Source: three-view drawing plus pictorial views. Frame: mm from the lowest corner of the part. Give positions to 0.01 mm unless a question says otherwise; leave off trailing zeros. Write each loop counter-clockwise with the first axis right and the second up, starting at its lowest first coordinate (ties: lowest second). Pieces come first, ordered by that corner, then holes.
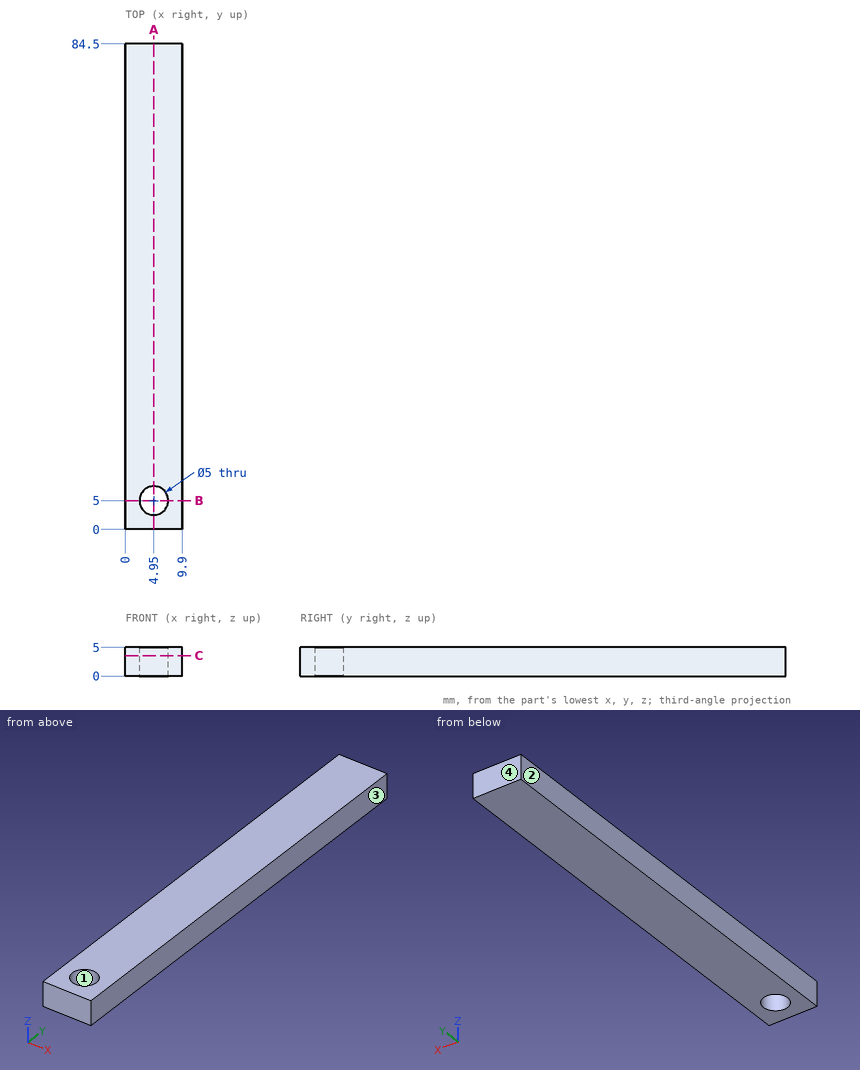
Q1. Ray query, line 1 along Y through (x, z) = (4.95, 1.1); line 2 along Y through (x, z) = (6.75, 3.9); line 3 along X through (y, z) = (6.5, 3.55). Return the intervals inside material, ascending.
Filled sheet:
line 1: y = 0 to 2.5, 7.5 to 84.5
line 2: y = 0 to 3.27, 6.73 to 84.5
line 3: x = 0 to 2.95, 6.95 to 9.9
Q2. Pin query (flat end, axial travel): P1, Ø1.5, axis at x = 7, y = 43.5, coming from the -Z side; P2, Ø4, axis at x = 4.95, y = 5, coming from the -Z side. Return the tip coordinate at first contact, or that it passes through.
Filled sheet:
P1: stops at z = 0
P2: passes through
Q3. Section B-B on y = 5. Output: boundary loops of the cut face in (x, z), plus the area to 3 significant figures.
Filled sheet:
outline: (0, 0) - (2.45, 0) - (2.45, 5) - (0, 5) - close; (7.45, 0) - (9.9, 0) - (9.9, 5) - (7.45, 5) - close
area: 24.5 mm2
Q4. Pull-direction query (X, two-part tool) for the marked faces 1, 2, 3 and 4; classes: released by +X, released by -X, zero draft, split by the parting line, or undercut.
Filled sheet:
face 1: undercut
face 2: released by -X
face 3: released by +X
face 4: zero draft
Q5. Section C-C on z = 3.55. Output: boundary loops of the cut face in (x, y), plus the area to 3 significant figures.
Filled sheet:
outline: (0, 0) - (9.9, 0) - (9.9, 84.5) - (0, 84.5) - close; hole circle Ø5 at (4.95, 5)
area: 817 mm2
Q6. Section A-A on x = 4.95. Output: boundary loops of the cut face in (y, z), plus the area to 4 significant figures.
Filled sheet:
outline: (0, 0) - (2.5, 0) - (2.5, 5) - (0, 5) - close; (7.5, 0) - (84.5, 0) - (84.5, 5) - (7.5, 5) - close
area: 397.5 mm2
